Can you work these out from the model? Positions are in its coordinate system, mm. Face numbers are marked on the shaded views. A direction names the side the tool comes from. Round coordinates to 2 decimals unless told otherwise and drop trailing zeros. Order: outer loops, then holes, each group sorted by start corner. A loop starts at its lowest first (then second) coordinate and runs counter-clockwise, first axis right, second up.
Q1. Will these pins go through, and if not, where does the flat tip stop? P1, Ø1.5, axis at y = 9.19, z = -9.19, coming from the -X side; P2, Ø5, axis at x = 93, z = -9.5, coming from the -Y side; P3, Ø2, axis at y = -12.5, z = 2.5, coming from the -X side.
Q2. If we section it at D-D (x = 43): Please give me the cut outline in (y, z).
Q3. For the marked faces 1, 2 and 3, which set-ups out of +Z, -Z, +X, -X, +Y, -Y let a thin tool reach every point of the face, with its end or its side?
Q4. If I drill on line 1 (Y direction, x = 5, z = 2.5); line 2 (Y direction, x = 80.5, z = -12); line 3 (X direction, y = 3, z = 4.5), over which ranges is the centre line in solid material (lowest first)?
Q5. If we section it at A-A (y = 0): Please give me the cut outline in (x, z), plus the area to 3 significant figures.
Q6. If we section it at C-C (x = 74): Please give me the cut outline in (y, z).
Q7. If we section it at B-B (z = 0): Please give me the cut outline in (x, y).
from build123d import *

# Parameters (mm, degrees)
CUT_EXTRUDE1_DEPTH        = 117.125836918
CUT_EXTRUDE1_DEPTH_BACK   = 117.125836918
SKETCH2_W                 = 12
SKETCH2_H                 = 0.5
CHAMFER1_SIZE             = 0.25
SKETCH3_W                 = 20
SKETCH3_H                 = 2
CUT_EXTRUDE2_DEPTH        = 3
M3X0_5_TAPPED_HOLE1_D     = 2.5
M3X0_5_TAPPED_HOLE1_DEPTH = 5.5
M3X0_5_TAPPED_HOLE1_TIP   = 0.751075774


with BuildPart() as part:
    # Sketch1 → Revolve1 (revolve)
    with BuildSketch(Plane(origin=(0, 0, 0), x_dir=(1, 0, 0), z_dir=(0, 1, 0)), mode=Mode.PRIVATE) as revolve1_sk:
        Polygon((0, 0), (113.9, 0), (113.9, 1.5), (106.9, 1.5), (106.9, 15), (60.3, 15), (60.3, 16), (19.3, 16), (19.3, 10), (16.3, 10), (16.3, 3), (0, 3), align=None)
    revolve(revolve1_sk.sketch.rotate(Axis((0, 0, 0), (1, 0, 0)), 180), axis=Axis((0, 0, 0), (1, 0, 0)))

    # Sketch2 → Cut-Extrude1 (cut, two sides: drawn at the far end of the back side and taken through both)
    with BuildSketch(Plane(origin=(0, 0, 0), x_dir=(1, 0, 0), z_dir=(0, 1, 0)).offset(-CUT_EXTRUDE1_DEPTH_BACK)):
        with Locations((6, 2.75)):
            Rectangle(SKETCH2_W, SKETCH2_H)
    extrude(amount=CUT_EXTRUDE1_DEPTH + CUT_EXTRUDE1_DEPTH_BACK, mode=Mode.SUBTRACT)

    # Chamfer1
    chamfer1_edges = [part.edges().sort_by_distance(p)[0] for p in [
        (19.3, 0, -16),
        (0, 2.872281323, 0.866025404),
    ]]
    chamfer(chamfer1_edges, length=CHAMFER1_SIZE)

    # Sketch3 → Cut-Extrude2 (cut)
    with BuildSketch(Plane.ZY.offset(-16.3)):
        with Locations((0, 10)):
            Rectangle(SKETCH3_W, SKETCH3_H)
        with Locations((0, -10)):
            Rectangle(SKETCH3_W, SKETCH3_H)
    extrude(amount=-CUT_EXTRUDE2_DEPTH, mode=Mode.SUBTRACT)

    # M3x0.5 Tapped Hole1
    with Locations(Plane.ZY.offset(-19.3)):
        with Locations((-9.192388155, -9.192388155), (-9.192388155, 9.192388155), (9.192388155, 9.192388155), (9.192388155, -9.192388155)):
            Hole(M3X0_5_TAPPED_HOLE1_D / 2, depth=M3X0_5_TAPPED_HOLE1_DEPTH)
            with Locations((0, 0, -(M3X0_5_TAPPED_HOLE1_DEPTH + M3X0_5_TAPPED_HOLE1_TIP / 2))):  # 118° drill point
                Cone(0, M3X0_5_TAPPED_HOLE1_D / 2, M3X0_5_TAPPED_HOLE1_TIP, mode=Mode.SUBTRACT)


solid = part.part
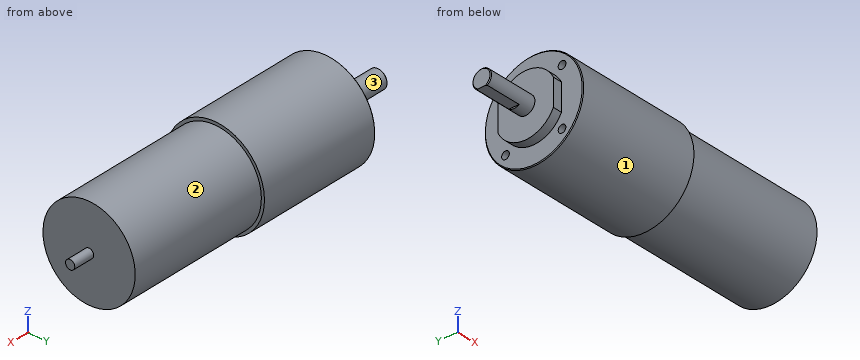
Solution:
1. P1: stops at x = 25.1
1. P2: stops at y = -13.27
1. P3: stops at x = 19.3
2. outline: circle Ø32 at (0, 0)
3. face 1: +X, -X
3. face 2: +X
3. face 3: -X
4. line 1: y = -1.66 to 1.66
4. line 2: y = -9 to 9
4. line 3: x = 16.3 to 106.9
5. outline: (0, -2.5) - (12, -2.5) - (12, -3) - (16.3, -3) - (16.3, -10) - (19.3, -10) - (19.3, -15.75) - (19.55, -16) - (60.3, -16) - (60.3, -15) - (106.9, -15) - (106.9, -1.5) - (113.9, -1.5) - (113.9, 1.5) - (106.9, 1.5) - (106.9, 15) - (60.3, 15) - (60.3, 16) - (19.55, 16) - (19.3, 15.75) - (19.3, 10) - (16.3, 10) - (16.3, 3) - (0.25, 3) - (0, 2.75) - close
5. area: 2,880 mm2
6. outline: circle Ø30 at (0, 0)
7. outline: (0, -2.75) - (0.25, -3) - (16.3, -3) - (16.3, -9) - (19.3, -9) - (19.3, -15.75) - (19.55, -16) - (60.3, -16) - (60.3, -15) - (106.9, -15) - (106.9, -1.5) - (113.9, -1.5) - (113.9, 1.5) - (106.9, 1.5) - (106.9, 15) - (60.3, 15) - (60.3, 16) - (19.55, 16) - (19.3, 15.75) - (19.3, 9) - (16.3, 9) - (16.3, 3) - (0.25, 3) - (0, 2.75) - close
